Model file for the job. Use its own axes, mm. Face numbers are marked on the shaded views. A direction names the side the tool comes from. Round coordinates to 2 decimals unless told otherwise and drop trailing zeros. Loops run counter-clockwise (first coordinate to the right, second up) from the corner with the lowest first, then second, coordinate; pieces in that order, holes last. Notation, with made-up numbers: M 43,-3.75 L 70,-3.75 A17 cw 70,20.25 Z; hole C -13,-22.5 d6. An arc over 180 degrees is marked long. Use a Markdown table: item, result. Add a question column.
Q1. Tool access for the marked faces 1, 2 and 3: list every direction of +Z, -Z, +X, -X, +Y, -Y with a clear straight run to the whole face (end or side of a thin tool).
Q2. Mould opens along Y. For the marked faces 4, 5 and 6 say: +Y half, -Y half, draft (parallel to the pull), parting line (faces both ways), or undercut.
Q3. Cut at C-C (y = 48). Give the cut face in (x, z).
Q4. Probe line 1 (Y direction, x = -16, z = 4); line 2 (Y direction, x = 29.5, z = 7.5); line 3 (Y direction, x = 41, z = 2.5). List the from-to ranges inside material, lowest first. Write a range as from..to.
Q5. Cut at B-B (x = -28.5). Give the cut face in (y, z), plus the area to 3 significant figures.
Q6. Pin check, flat tips, straight feed: pin 1 (4 mm diameter, centred on y = 33.5, z = 3, fed in from +X); pin 2 (2 mm diameter, centred on y = 30, z = 2.5, fed in from +X); pin 3 (1.8 mm diameter, centred on x = -42.5, z = 5, fed in from -Y). Stop position of each tip, or through.
Q7. Cut at A-A (z = 5). Give the cut face in (x, y).
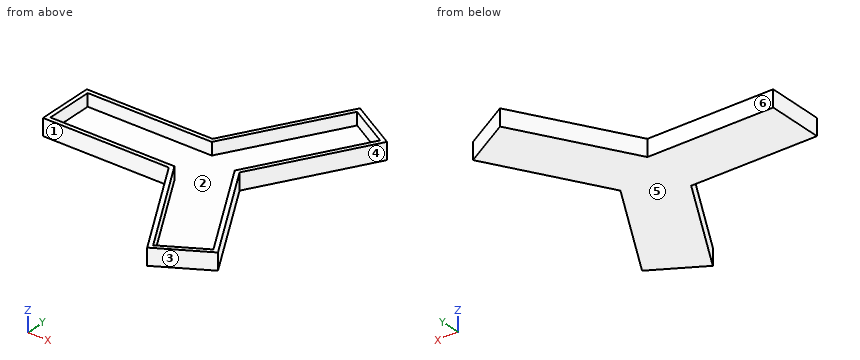
from build123d import *

# Parameters (mm, degrees)
PAD002_DEPTH = 8
PAD_DEPTH    = 2
ARRAY_COUNT  = 3


with BuildPart() as pad002:
    # Sketch002 → Pad002 (new body)
    with BuildSketch(Plane.XY):
        Polygon((-6.6395280957, 11.5), (-7.7942286341, 13.5), (-68, 13.5), (-68, -13.5), (-7.7942286341, -13.5), (-6.6395280957, -11.5), (-66, -11.5), (-66, 11.5), align=None)
    extrude(amount=PAD002_DEPTH)


with BuildPart() as array:
    # Sketch → Pad (new body)
    with BuildSketch(Plane.XY):
        Polygon((0, 0), (-7.7942286341, 13.5), (-68, 13.5), (-68, -13.5), (-7.7942286341, -13.5), align=None)
    extrude(amount=PAD_DEPTH)

    # Fusion: union Pad002
    add(pad002.part)

    # Array: Array ×3 about axis
    array_axis = Axis((0, 0, 0), (0, 0, 1))


with BuildPart() as array_1:
    add(array.part)
    for i in range(1, ARRAY_COUNT):
        add(array.part.rotate(array_axis, i * 360 / ARRAY_COUNT))


solid = array_1.part
Checked values:
| question | item | result |
|---|---|---|
| 1 | face 1 | +Z, -Z, -X, -Y |
| 1 | face 2 | +Z |
| 1 | face 3 | +Z, -Z, +X, -Y |
| 2 | face 4 | undercut |
| 2 | face 5 | draft |
| 2 | face 6 | +Y half |
| 3 | outline | M 12.12,0 L 43.3,0 L 43.3,8 L 40.99,8 L 40.99,2 L 14.43,2 L 14.43,8 L 12.12,8 Z |
| 4 | line 1 | y = -13.5..-11.5, 11.5..13.5 |
| 4 | line 2 | y = -61.49..-59.18, -28.1..-24.1, 24.1..28.1, 59.18..61.49 |
| 4 | line 3 | y = -54.85..-52.54, -48.01..-44.01, 44.01..48.01, 52.54..54.85 |
| 5 | outline | M -13.5,0 L 13.5,0 L 13.5,8 L 11.5,8 L 11.5,2 L -11.5,2 L -11.5,8 L -13.5,8 Z |
| 5 | area | 78.0 mm^2 |
| 6 | pin 1 | stops at x = 36.08 |
| 6 | pin 2 | stops at x = 33.49 |
| 6 | pin 3 | stops at y = -13.5 |
| 7 | outline | M -68,-13.5 L -7.79,-13.5 L 22.31,-65.64 L 45.69,-52.14 L 15.59,0 L 45.69,52.14 L 22.31,65.64 L -7.79,13.5 L -68,13.5 Z; hole M -66,-11.5 L -6.64,-11.5 L 23.04,-62.91 L 42.96,-51.41 L 13.28,0 L 42.96,51.41 L 23.04,62.91 L -6.64,11.5 L -66,11.5 Z |
